```python
from build123d import *

# Parameters (mm, degrees)
SKETCH2_W           = 177.8
SKETCH2_H           = 101.6
BOSS_EXTRUDE3_DEPTH = 6.35
SKETCH3_R           = 10.95
SKETCH3_R_2         = 3.175
SKETCH3_R_3         = 7
CUT_EXTRUDE1_DEPTH  = 103.587389576
SKETCH7_W           = 14
SKETCH7_H           = 6.35
SKETCH7_W_2         = 6.35
SKETCH7_H_2         = 14
SKETCH7_W_3         = 5.08
SKETCH7_H_3         = 101.6
CUT_EXTRUDE2_DEPTH  = 103.587389576
SKETCH8_W           = 5
SKETCH8_H           = 3
SKETCH8_W_2         = 4.987190998
SKETCH8_R           = 2.65
CUT_EXTRUDE3_DEPTH  = 103.587389576


with BuildPart() as part:
    # Sketch2 → Boss-Extrude3 (new body)
    with BuildSketch(Plane.XY):
        Rectangle(SKETCH2_W, SKETCH2_H)
    extrude(amount=BOSS_EXTRUDE3_DEPTH)

    # Sketch3 → Cut-Extrude1 (cut, through all)
    with BuildSketch(Plane.XY.offset(6.35)):
        with Locations((-9.4120506, 0)):
            Circle(SKETCH3_R)
        with Locations((-42.64375, 0)):
            Circle(SKETCH3_R_2)
        with Locations((-66.216922318, 23.573172318)):
            Circle(SKETCH3_R_3)
        with Locations((-19.070577682, 23.573172318)):
            Circle(SKETCH3_R_3)
        with Locations((-66.216922318, -23.573172318)):
            Circle(SKETCH3_R_3)
        with Locations((-19.070577682, -23.573172318)):
            Circle(SKETCH3_R_3)
        with Locations((45.9739194, 0)):
            Circle(SKETCH3_R)
    extrude(amount=-CUT_EXTRUDE1_DEPTH, mode=Mode.SUBTRACT)

    # Sketch7 → Cut-Extrude2 (cut, through all)
    with BuildSketch(Plane.XY.offset(6.35)):
        with Locations((63.509, -47.625)):
            Rectangle(SKETCH7_W, SKETCH7_H)
        with Locations((63.509, 47.625)):
            Rectangle(SKETCH7_W, SKETCH7_H)
        with Locations((0, 47.625)):
            Rectangle(SKETCH7_W, SKETCH7_H)
        with Locations((0, -47.625)):
            Rectangle(SKETCH7_W, SKETCH7_H)
        Polygon((-82.55, -38.1), (-88.9, -38.1), (-88.9, -44.45), (-88.9, -50.8), (-74.9, -50.8), (-74.9, -44.45), (-82.55, -44.45), align=None)
        with Locations((-85.725, 0)):
            Rectangle(SKETCH7_W_2, SKETCH7_H_2)
        Polygon((-88.9, 44.45), (-88.9, 38.1), (-82.55, 38.1), (-82.55, 44.45), (-74.9, 44.45), (-74.9, 50.8), (-88.9, 50.8), align=None)
        with Locations((86.36, 0)):
            Rectangle(SKETCH7_W_3, SKETCH7_H_3)
    extrude(amount=-CUT_EXTRUDE2_DEPTH, mode=Mode.SUBTRACT)

    # Sketch8 → Cut-Extrude3 (cut, through all)
    with BuildSketch(Plane(origin=(0, 0, 0), x_dir=(-1, 0, 0), z_dir=(0, 0, -1))):
        with Locations((-61.809, -26.465)):
            Rectangle(SKETCH8_W, SKETCH8_H)
        Polygon((-59.321809002, -30.694855507), (-64.321809002, -30.694855507), (-64.309, -34.215), (-59.309, -34.215), align=None)
        with Locations((-33.689, -26.465)):
            Rectangle(SKETCH8_W, SKETCH8_H)
        with Locations((-43.143748621, -41.147)):
            Rectangle(SKETCH8_W, SKETCH8_H)
        with Locations((-43.143748621, -34.897)):
            Rectangle(SKETCH8_W, SKETCH8_H)
        with Locations((-33.695404501, -32.715)):
            Rectangle(SKETCH8_W_2, SKETCH8_H)
        with Locations((-43.143748621, 41.147)):
            Rectangle(SKETCH8_W, SKETCH8_H)
        with Locations((-43.143748621, 34.897)):
            Rectangle(SKETCH8_W, SKETCH8_H)
        with Locations((-33.701809002, 32.715)):
            Rectangle(SKETCH8_W, SKETCH8_H)
        with Locations((-33.701809002, 26.465)):
            Rectangle(SKETCH8_W, SKETCH8_H)
        with Locations((-72.850352522, 40.626855507)):
            Rectangle(SKETCH8_W, SKETCH8_H)
        with Locations((-72.850352522, 34.376855507)):
            Rectangle(SKETCH8_W, SKETCH8_H)
        with Locations((-61.821809002, 32.194855507)):
            Rectangle(SKETCH8_W, SKETCH8_H)
        with Locations((-61.821809002, 25.944855507)):
            Rectangle(SKETCH8_W, SKETCH8_H)
        with Locations((-72.850352522, -34.376855507)):
            Rectangle(SKETCH8_W, SKETCH8_H)
        with Locations((-72.850352522, -40.626855507)):
            Rectangle(SKETCH8_W, SKETCH8_H)
        with Locations((-80.320280368, 38.022017825)):
            Circle(SKETCH8_R)
        with Locations((-80.167417552, -38.111532033)):
            Circle(SKETCH8_R)
    extrude(amount=-CUT_EXTRUDE3_DEPTH, mode=Mode.SUBTRACT)


solid = part.part
```
Geometry: final body of the model. Coordinates: model frame, mm. A direction names the side the tool comes from. Coordinates: 2 decimals unless noted, no trailing zeros. Loops run counter-clockwise (first coordinate to the right, second up) from the corner with the lowest first, then second, coordinate; pieces in that order, holes last. Notation, with made-up numbers: M 23.25,62 L 48.25,62 A19 cw 48.25,85 Z; hole C 19,-8 d5. An arc over 180 degrees is marked long. Put each result on its own line as item: value.
(1) Cut plane D-D on z = 4.5. State how many separate pieces and enclosed holes the cut face has, then the cut area to 3 significant figures.
Answer sheet:
separate pieces: 1
enclosed holes: 25
area: 15,200 mm^2
(2) Cut plane B-B on x = 61. Return the cut outline in (y, z) (3 decimals), then the cut area to 3 significant figures.
Answer sheet:
outline: M -44.45,0 L -34.215,0 L -34.215,6.35 L -44.45,6.35 Z; M -30.695,0 L -27.965,0 L -27.965,6.35 L -30.695,6.35 Z; M -24.965,0 L 24.445,0 L 24.445,6.35 L -24.965,6.35 Z; M 27.445,0 L 30.695,0 L 30.695,6.35 L 27.445,6.35 Z; M 33.695,0 L 44.45,0 L 44.45,6.35 L 33.695,6.35 Z
area: 485 mm^2
(3) Cut plane A-A on y = 0. Return the cut outline in (x, z).
Answer sheet:
outline: M -82.55,0 L -45.82,0 L -45.82,6.35 L -82.55,6.35 Z; M -39.47,0 L -20.36,0 L -20.36,6.35 L -39.47,6.35 Z; M 1.54,0 L 35.02,0 L 35.02,6.35 L 1.54,6.35 Z; M 56.92,0 L 83.82,0 L 83.82,6.35 L 56.92,6.35 Z
(4) Material intervals for probe 1 along Y at (x, z) = (62, 3) (3 decimals); probe 2 along X at (y, z) = (-32, 6.25); probe 3 along X at (y, z) = (35, 3.5), sorted ascending.
Answer sheet:
probe 1: y = -44.45 to -34.215, -30.695 to -27.965, -24.965 to 24.445, 27.445 to 30.695, 33.695 to 44.45
probe 2: x = -88.9 to 31.2, 36.19 to 59.32, 64.32 to 83.82
probe 3: x = -88.9 to 40.64, 45.64 to 70.35, 75.35 to 83.82
(5) Access query for faces 4 (the face through (73, -35.877, 3)), 5 (the face through (56.509, -48, 3)), 6 (the face through (56.509, 48, 3)), 7 (the face through (-82.55, 41, 3)), 8 (the face through (-82.55, -41, 3)). Directions: +Z, -Z, +X, -X, +Y, -Y. A direction counts if a zero-diameter tool reaches every point of the face in a straight line with its end or side. Return the directions, or none.
Answer sheet:
face 4: +Z, -Z
face 5: +Z, -Z, -Y
face 6: +Z, -Z, +Y
face 7: +Z, -Z, -X, +Y
face 8: +Z, -Z, -X, -Y
(6) First-contact query: pin 1 (2.5 mm diameter, centred on x = 63, z = 3, fed in from +Y); pin 2 (11 mm diameter, centred on x = -66.22, y = 23.57, fed in from -Z); pin 3 (1.9 mm diameter, centred on y = -46, z = 4.5, fed in from -X). Flat tips, straight axial feed; report the tip coordinate or a pass-through.
Answer sheet:
pin 1: stops at y = 44.45
pin 2: passes through
pin 3: stops at x = -74.9
(7) Draft query along X for faces 1 (the face through (83.82, -1, 3)), 2 (the face through (43, 39.647, 3)), 3 (the face through (-82.55, 0, 3)). Return one class per face: pulls with the +X half, pulls with the -X half, needs draft (parallel to the pull), parting line crosses it, or undercut.
Answer sheet:
face 1: pulls with the +X half
face 2: undercut
face 3: pulls with the -X half
(8) Cut plane C-C on x = -23. Return the cut outline in (y, z).
Answer sheet:
outline: M -50.8,0 L -29.37,0 L -29.37,6.35 L -50.8,6.35 Z; M -17.78,0 L 17.78,0 L 17.78,6.35 L -17.78,6.35 Z; M 29.37,0 L 50.8,0 L 50.8,6.35 L 29.37,6.35 Z
